Geometry check sheet. Reference: the model listing, model coordinates, mm. Face numbers are marked on the shaded views. A direction names the side the tool comes from. Round coordinates to 2 decimals unless told otherwise and drop trailing zeros. Order: outer loops, then holes, each group sorted by start corner. A loop starts at its lowest first (then second) coordinate and runs counter-clockwise, first axis right, second up.
(1) Sectioned sample at A-A (y = 14). Record the boundary of the cut face in (x, z) (3 decimals).
(2) Release check for a two-part mould opening along Y. For the marked faces 3, 4, 5 and 6 record: +Y half, -Y half, draft (parallel to the pull), parting line (faces both ways), or undercut.
(3) Sectioned sample at C-C (x = 27.5). Record the boundary of the cut face in (y, z) (3 decimals).
(4) Material ranges on line 1 along X through (y, z) = (14, 7.25) (3 decimals); line 2 along Y through (x, z) = (41, 15.25) (3 decimals); line 3 along Z through (x, y) = (9.5, 15) (3 decimals), recorded low to high.
(5) Go/stop test with flat-tipped pins: pin 1 (8 mm diameter, centred on x = 16, z = 9, fed in from -Y); pin 2 (1 mm diameter, centred on x = 1.5, y = 11, fed in from -Z) (3 decimals); pin 3 (1 mm diameter, centred on x = 24, y = 9.5, fed in from -Z) (3 decimals). Record where each tip stops, or that it passes through.
(6) Set-up check for the marked faces 1 and 2: record each of +Z, -Z, +X, -X, +Y, -Y from which the full face is reachable in a straight line by a thin tool's end or side.
(7) Sectioned sample at B-B (z = 8.5). Record the boundary of the cut face in (x, y) (3 decimals).
from build123d import *

# Parameters (mm, degrees)
SKETCH1_W           = 44.45
SKETCH1_H           = 38.1
BOSS_EXTRUDE1_DEPTH = 25.4
SKETCH2_W           = 38.1
SKETCH2_H           = 31.75
CUT_EXTRUDE1_DEPTH  = 22.225
SKETCH3_R           = 3.175
SKETCH3_R_2         = 1.5875
CUT_EXTRUDE2_DEPTH  = 22.225
CUT_EXTRUDE3_DEPTH  = 3.175


with BuildPart() as part:
    # Sketch1 → Boss-Extrude1 (new body)
    with BuildSketch(Plane.XY):
        with Locations((22.225, 19.05)):
            Rectangle(SKETCH1_W, SKETCH1_H)
    extrude(amount=BOSS_EXTRUDE1_DEPTH)

    # Sketch2 → Cut-Extrude1 (cut)
    with BuildSketch(Plane(origin=(0, 0, 0), x_dir=(-1, 0, 0), z_dir=(0, 0, -1))):
        with Locations((-22.225, 19.05)):
            Rectangle(SKETCH2_W, SKETCH2_H)
    extrude(amount=-CUT_EXTRUDE1_DEPTH, mode=Mode.SUBTRACT)

    # Sketch3 → Cut-Extrude2 (cut)
    with BuildSketch(Plane.XY.offset(25.4)):
        with Locations((22.225, 27.78125)):
            Circle(SKETCH3_R)
        with Locations((22.225, 10.31875)):
            Circle(SKETCH3_R_2)
    extrude(amount=-CUT_EXTRUDE2_DEPTH, mode=Mode.SUBTRACT)

    # Sketch4 → Cut-Extrude3 (cut)
    with BuildSketch(Plane(origin=(0, 0, 0), x_dir=(-1, 0, 0), z_dir=(0, 0, -1))):
        Polygon((-41.275, 26.51125), (-41.275, 29.05125), (-44.45, 30.32125), (-44.45, 25.24125), align=None)
        Polygon((-44.45, 12.85875), (-41.275, 11.58875), (-41.275, 9.04875), (-44.45, 7.77875), align=None)
        Polygon((0, 25.24125), (-3.175, 26.51125), (-3.175, 29.05125), (0, 30.32125), align=None)
        Polygon((0, 12.85875), (0, 7.77875), (-3.175, 9.04875), (-3.175, 11.58875), align=None)
    extrude(amount=-CUT_EXTRUDE3_DEPTH, mode=Mode.SUBTRACT)


solid = part.part
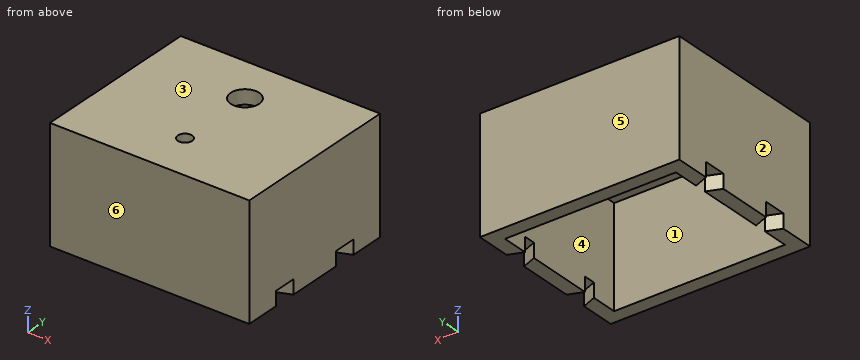
Answer below:
1. outline: (0, 0) - (3.175, 0) - (3.175, 22.225) - (41.275, 22.225) - (41.275, 0) - (44.45, 0) - (44.45, 25.4) - (0, 25.4) - close
2. face 3: draft
2. face 4: undercut
2. face 5: +Y half
2. face 6: -Y half
3. outline: (0, 0) - (3.175, 0) - (3.175, 22.225) - (34.925, 22.225) - (34.925, 0) - (38.1, 0) - (38.1, 25.4) - (0, 25.4) - close
4. line 1: x = 0 to 3.175, 41.275 to 44.45
4. line 2: y = 0 to 3.175, 34.925 to 38.1
4. line 3: z = 22.225 to 25.4
5. pin 1: stops at y = 0
5. pin 2: stops at z = 3.175
5. pin 3: stops at z = 22.225
6. face 1: -Z
6. face 2: +Z, -Z, -X, +Y, -Y
7. outline: (0, 0) - (44.45, 0) - (44.45, 38.1) - (0, 38.1) - close; hole (3.175, 3.175) - (41.275, 3.175) - (41.275, 34.925) - (3.175, 34.925) - close
